from build123d import *

# Parameters (mm, degrees)
SKETCH1_W           = 30
SKETCH1_H           = 15
BOSS_EXTRUDE1_DEPTH = 15
CUT_EXTRUDE1_DEPTH  = 23.5


with BuildPart() as part:
    # Sketch1 → Boss-Extrude1 (new body)
    with BuildSketch(Plane(origin=(0, 0, 0), x_dir=(1, 0, 0), z_dir=(0, 1, 0))):
        Rectangle(SKETCH1_W, SKETCH1_H)
    extrude(amount=BOSS_EXTRUDE1_DEPTH)

    # Sketch2 → Cut-Extrude1 (cut, through all)
    with BuildSketch(Plane(origin=(0, 15, 0), x_dir=(1, 0, 0), z_dir=(0, 1, 0))):
        with BuildLine():
            Line((-10.3, 0), (-9.424773748, -1.363692694))
            ThreePointArc((-9.424773748, -1.363692694), (-7.3, 0), (-9.424773748, 1.363692694))
            Line((-9.424773748, 1.363692694), (-10.3, 0))
        make_face()
        with BuildLine():
            Line((-2.6, 0), (-1.195098007, -2.309056248))
            ThreePointArc((-1.195098007, -2.309056248), (2.6, 0), (-1.195098007, 2.309056248))
            Line((-1.195098007, 2.309056248), (-2.6, 0))
        make_face()
        with BuildLine():
            Line((7.3, 0), (8.175226252, -1.363692694))
            ThreePointArc((8.175226252, -1.363692694), (10.3, 0), (8.175226252, 1.363692694))
            Line((8.175226252, 1.363692694), (7.3, 0))
        make_face()
    extrude(amount=-CUT_EXTRUDE1_DEPTH, mode=Mode.SUBTRACT)


solid = part.part
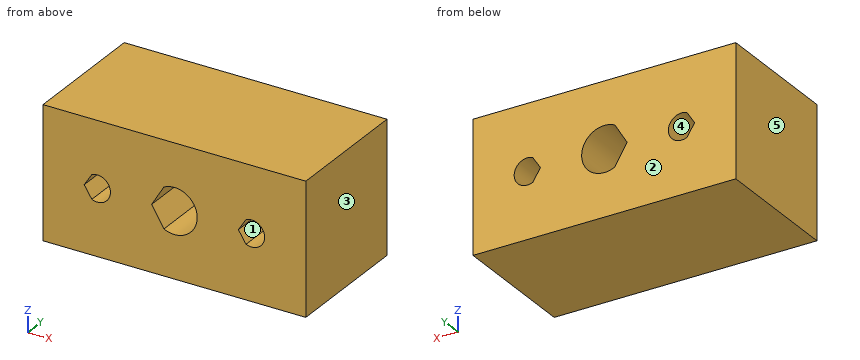
Part model, mm, in its own coordinate system. Face numbers are marked on the shaded views. A direction names the side the tool comes from. Coordinates: 2 decimals unless noted, no trailing zeros. Order: outer loops, then holes, each group sorted by start corner. A loop starts at its lowest first (then second) coordinate and runs counter-clockwise, first axis right, second up.
(1) Slice it at B-B, the plane z = -2. Write the cut outline in (x, y).
Check sheet entries:
outline: (-15, 0) - (-1.38, 0) - (-1.38, 15) - (-15, 15) - close; (1.66, 0) - (15, 0) - (15, 15) - (1.66, 15) - close
(2) Pin check, flat tip, straight feed: pin 1 Ø3 at (x, z) = (0, 0) entering from +Y. Stop position of the tip, or through.
Check sheet entries:
pin 1: passes through
(3) Tool access for the marked faces 1 and 2: list every direction of +Z, -Z, +X, -X, +Y, -Y with a clear straight run to the whole face (end or side of a thin tool).
Check sheet entries:
face 1: +Y, -Y
face 2: +Z, -Z, +X, -X, +Y
(4) Pull direction X, two halves, no side cores. Call the marked faces 3, 4 and 5: pulls with the +X half, pulls with the -X half, needs draft (parallel to the pull), parting line crosses it, or undercut.
Check sheet entries:
face 3: pulls with the +X half
face 4: undercut
face 5: pulls with the -X half
(5) Slice it at A-A, the plane x = 0. Write the cut outline in (y, z), and give its area (3 significant figures).
Check sheet entries:
outline: (0, -7.5) - (15, -7.5) - (15, -2.6) - (0, -2.6) - close; (0, 2.6) - (15, 2.6) - (15, 7.5) - (0, 7.5) - close
area: 147 mm2
(6) Slice it at C-C, the plane y = 12.25. Write the cut outline in (x, z), and give its area (3 significant figures).
Check sheet entries:
outline: (-15, -7.5) - (15, -7.5) - (15, 7.5) - (-15, 7.5) - close; hole (-10.3, 0) - (-9.42, -1.36) arc R1.5 ccw (long way) to (-9.42, 1.36) - close; hole (-2.6, 0) - (-1.2, -2.31) arc R2.6 ccw (long way) to (-1.2, 2.31) - close; hole (7.3, 0) - (8.18, -1.36) arc R1.5 ccw (long way) to (8.18, 1.36) - close
area: 417 mm2
(7) Probe L1, parallel to Z at x = -8.8, y = 12; L2, parallel to X at y = 10.25, z = -0.5; L3, parallel to Z at x = -1.25, y = 7. List the from-to ranges inside material, lowest first.
Check sheet entries:
L1: z = -7.5 to -1.5, 1.5 to 7.5
L2: x = -15 to -9.98, -7.39 to -2.3, 2.55 to 7.62, 10.21 to 15
L3: z = -7.5 to -2.22, 2.22 to 7.5
